from build123d import *

# Parameters (mm, degrees)
EXTRUDE_1_DEPTH     = 10
FILLET_1_R          = 5
SKETCH_2_W          = 14.503098638
SKETCH_2_H          = 45
EXTRUDE_4_DEPTH     = 10
FILLET_3_R          = 5
SKETCH_3_R          = 5
CUT_EXTRUDE_2_DEPTH = 82.929848041
FILLET_4_R          = 5
SKETCH_4_R          = 5
CUT_EXTRUDE_5_DEPTH = 70.372184628
EXTRUDE_7_DEPTH     = 10


with BuildPart() as part:
    # 草图1 → 凸台-拉伸1 (new body)
    with BuildSketch(Plane.XY):
        Polygon((37.5, 57.5), (-37.5, 57.5), (-37.5, 32.5), (-5, 0), (-37.5, -32.5), (-37.5, -57.5), (37.5, -57.5), align=None)
    extrude(amount=EXTRUDE_1_DEPTH)

    # 圆角1
    fillet_1_edges = [part.edges().sort_by_distance(p)[0] for p in [
        (-5, 0, 5),
        (-37.5, 32.5, 5),
        (-37.5, -32.5, 5),
    ]]
    fillet(fillet_1_edges, radius=FILLET_1_R)

    # 草图2 → 凸台-拉伸4 (add)
    with BuildSketch(Plane.XY.offset(10)):
        Polygon((37.5, 57.5), (37.5, 0), (42.996901362, 0), (42.996901362, 45), (57.5, 45), align=None)
        with Locations((50.248450681, 22.5)):
            Rectangle(SKETCH_2_W, SKETCH_2_H)
        with Locations((50.248450681, -22.5)):
            Rectangle(SKETCH_2_W, SKETCH_2_H)
        Polygon((37.5, 0), (37.5, -57.5), (57.5, -45), (42.996901362, -45), (42.996901362, 0), align=None)
    extrude(amount=-EXTRUDE_4_DEPTH)

    # 圆角3
    fillet_3_edges = [part.edges().sort_by_distance(p)[0] for p in [
        (57.5, -45, 5),
        (57.5, 45, 5),
    ]]
    fillet(fillet_3_edges, radius=FILLET_3_R)

    # 草图3 → 切除-拉伸2 (cut, through all)
    with BuildSketch(Plane.XY.offset(10)):
        Polygon((17.5, 57.5), (37.5, 45), (37.5, 57.5), align=None)
        with BuildLine():
            Line((37.5, 57.5), (37.5, -57.5))
            Line((37.5, -57.5), (55.1499947, -46.468753312))
            ThreePointArc((55.1499947, -46.468753312), (56.873212406, -44.652604454), (57.5, -42.228761792))
            Line((57.5, -42.228761792), (57.5, 42.228761792))
            ThreePointArc((57.5, 42.228761792), (56.873212406, 44.652604454), (55.1499947, 46.468753312))
            Line((55.1499947, 46.468753312), (37.5, 57.5))
        make_face()
        Polygon((37.5, -45), (17.5, -57.5), (37.5, -57.5), align=None)
        with Locations((4.5, -32.5)):
            Circle(SKETCH_3_R)
        with Locations((4.5, 32.5)):
            Circle(SKETCH_3_R)
    extrude(amount=-CUT_EXTRUDE_2_DEPTH, mode=Mode.SUBTRACT)

    # 圆角4
    fillet_4_edges = [part.edges().sort_by_distance(p)[0] for p in [
        (37.5, -45, 5),
        (37.5, 45, 5),
    ]]
    fillet(fillet_4_edges, radius=FILLET_4_R)

    # 草图4 → 切除-拉伸5 (cut, through all)
    with BuildSketch(Plane.XY.offset(10)):
        with Locations((4.5, 40)):
            Circle(SKETCH_4_R)
        with Locations((4.5, 32.5)):
            Circle(SKETCH_4_R)
        with Locations((4.5, -40)):
            Circle(SKETCH_4_R)
        with Locations((4.5, -32.5)):
            Circle(SKETCH_4_R)
    extrude(amount=-CUT_EXTRUDE_5_DEPTH, mode=Mode.SUBTRACT)

    # 草图7 → 凸台-拉伸7 (add)
    with BuildSketch(Plane.XY.offset(10)):
        with BuildLine():
            ThreePointArc((1.192810861, 36.25), (2.442810861, 27.942810861), (9.5, 32.5))
            ThreePointArc((9.5, 32.5), (9.057189139, 34.557189139), (7.807189139, 36.25))
            ThreePointArc((7.807189139, 36.25), (4.5, 35), (1.192810861, 36.25))
        make_face()
        with BuildLine():
            ThreePointArc((7.807189139, -36.25), (9.057189139, -34.557189139), (9.5, -32.5))
            ThreePointArc((9.5, -32.5), (2.442810861, -27.942810861), (1.192810861, -36.25))
            ThreePointArc((1.192810861, -36.25), (4.5, -35), (7.807189139, -36.25))
        make_face()
    extrude(amount=-EXTRUDE_7_DEPTH)


solid = part.part
Source: CAD feature listing. Evaluate the final solid. Frame: model axes, mm. A direction names the side the tool comes from. Give positions to 0.01 mm unless a question says otherwise; leave off trailing zeros. Write each loop counter-clockwise with the first axis right and the second up, starting at its lowest first coordinate (ties: lowest second). Pieces come first, ordered by that corner, then holes. Notation, with made-up numbers: (-27, 50.5) -> (-13, 50.5) arc R19 ccw to (-13, 74.5) -> close; hole circle Ø4 at (-24, 43.25). An arc over 180 degrees is marked (long way). Return JSON: item names as keys, results as strings. Group by question number.
1. Section B-B, the plane x = -27. Output: boundary loops of the cut face in (y, z).
2. Access query for faces 1 (the face through (-37.5, -46, 5)), 2 (the face through (-22, -17, 5)). Directions: +Z, -Z, +X, -X, +Y, -Y. A direction counts if a zero-diameter tool reaches every point of the face in a straight line with its end or side. Return the directions, or none.
3. Material intervals for line 1 (Y direction, x = 3.5, z = 5.25); line 2 (X direction, y = -40, z = 5); line 3 (Y direction, x = 9, z = 5.75), sorted ascending. Write a range as from..to.
4. Section D-D, the plane x = 4.5. Output: boundary loops of the cut face in (y, z).
5. Mould query, pull axis Y, two halves, no side actions, for faces 3 (the face through (-1, 1, 10)), 4 (the face through (-37.11, -32.63, 5.07)), 5 (the face through (26.449, -51.907, 5.07)). Classes: +Y half, -Y half, draft (parallel to the pull), parting line (faces both ways), or undercut.
6. Section C-C, the plane z = 6.5. Output: boundary loops of the cut face in (x, y).
7. Section A-A, the plane y = 40. Output: boundary loops of the cut face in (x, z), then the cut area to 3 significant figures.
Determined:
{
 "1": {"outline": "(-57.5, 0) -> (-22, 0) -> (-22, 10) -> (-57.5, 10) -> close; (22, 0) -> (57.5, 0) -> (57.5, 10) -> (22, 10) -> close"},
 "2": {"face 1": "+Z, -Z, -X, +Y, -Y", "face 2": "+Z, -Z, -X"},
 "3": {"line 1": "y = -57.5..-44.9, -35.1..35.1, 44.9..57.5", "line 2": "x = -37.5..-0.5, 9.5..37.5", "line 3": "y = -57.5..-42.18, -37.82..37.82, 42.18..57.5"},
 "4": {"outline": "(-57.5, 0) -> (-45, 0) -> (-45, 10) -> (-57.5, 10) -> close; (-35, 0) -> (35, 0) -> (35, 10) -> (-35, 10) -> close; (45, 0) -> (57.5, 0) -> (57.5, 10) -> (45, 10) -> close"},
 "5": {"face 3": "draft", "face 4": "undercut", "face 5": "-Y half"},
 "6": {"outline": "(-37.5, -57.5) -> (17.5, -57.5) -> (35.15, -46.47) arc R5 ccw to (37.5, -42.23) -> (37.5, 42.23) arc R5 ccw to (35.15, 46.47) -> (17.5, 57.5) -> (-37.5, 57.5) -> (-37.5, 34.57) arc R5 ccw to (-36.04, 31.04) -> (-8.54, 3.54) arc R5 cw to (-8.54, -3.54) -> (-36.04, -31.04) arc R5 ccw to (-37.5, -34.57) -> close; hole circle Ø10 at (4.5, -40); hole circle Ø10 at (4.5, 40)"},
 "7": {"outline": "(-37.5, 0) -> (-0.5, 0) -> (-0.5, 10) -> (-37.5, 10) -> close; (9.5, 0) -> (37.5, 0) -> (37.5, 10) -> (9.5, 10) -> close", "area": "650 mm2"}
}
